```python
from build123d import *

# Parameters (mm, degrees)
SKETCH1_R           = 85
SKETCH1_R_2         = 65
SKETCH1_W           = 2.9
SKETCH1_H           = 40
BOSS_EXTRUDE1_DEPTH = 2.9


with BuildPart() as part:
    # Sketch1 → Boss-Extrude1 (new body)
    with BuildSketch(Plane.XY):
        Circle(SKETCH1_R)
        Circle(SKETCH1_R_2, mode=Mode.SUBTRACT)
        with Locations((-75, 0)):
            Rectangle(SKETCH1_W, SKETCH1_H, mode=Mode.SUBTRACT)
        with Locations((75, 0)):
            Rectangle(SKETCH1_W, SKETCH1_H, mode=Mode.SUBTRACT)
    extrude(amount=BOSS_EXTRUDE1_DEPTH)


solid = part.part
```
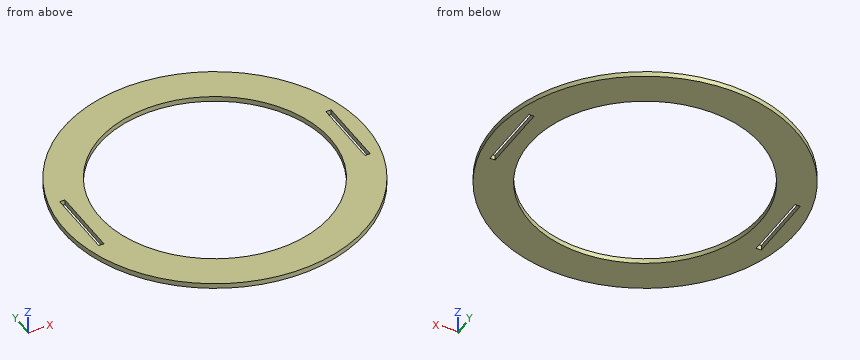
Build history of the part. All positions in model axes, mm. Give positions to 0.01 mm unless a question says otherwise; leave off trailing zeros. Order: outer loops, then holes, each group sorted by start corner. A loop starts at its lowest first (then second) coordinate and runs counter-clockwise, first axis right, second up. Notation, with made-up numbers: M -27,-39.75 L 29,-39.75 A29 cw 29,-6.75 Z; hole C 73.5,16.25 d5. An arc over 180 degrees is marked long. Write item = value, one per line. Start each with the question number.
(1) Pin check, flat tips, straight feed: pin 1 Ø1.5 at (x, z) = (6, 1) entering from -Y; pin 2 Ø0.9 at (y, z) = (-4.5, 2) entering from +X; pin 3 Ø0.9 at (x, z) = (-75.5, 1.5) entering from +Y; pin 4 Ø1.5 at (x, y) = (47.5, 58) entering from -Z. Stop position of each tip, or through.
(2) Probe L1, parallel to X at y = -1.5, z = 2.2; L2, parallel to Y at x = 0, z = 2.6; L3, parallel to Y at x = -59.5, z = 0.4. List the from-to ranges inside material, lowest first. Write a range as [from, to].
(3) Slice it at B-B on z = 2. Write the cut outline in (x, y), plus the area to 3 significant figures.
(4) Slice it at C-C on y = 0. Write the cut outline in (x, z).
(5) Slice it at D-D on y = 27.5. Write the cut outline in (x, z).
(6) Slice it at A-A on x = 0. Write the cut outline in (y, z).
Responses:
q1.pin_1 = -84.84
q1.pin_2 = 84.9
q1.pin_3 = 39.91
q1.pin_4 = 0
q2.L1 = [-84.99, -76.45], [-73.55, -64.98], [64.98, 73.55], [76.45, 84.99]
q2.L2 = [-85, -65], [65, 85]
q2.L3 = [-60.7, -26.17], [26.17, 60.7]
q3.outline = C 0,0 d170; hole M -76.45,-20 L -73.55,-20 L -73.55,20 L -76.45,20 Z; hole C 0,0 d130; hole M 73.55,-20 L 76.45,-20 L 76.45,20 L 73.55,20 Z
q3.area = 9,190 mm2
q4.outline = M -85,0 L -76.45,0 L -76.45,2.9 L -85,2.9 Z; M -73.55,0 L -65,0 L -65,2.9 L -73.55,2.9 Z; M 65,0 L 73.55,0 L 73.55,2.9 L 65,2.9 Z; M 76.45,0 L 85,0 L 85,2.9 L 76.45,2.9 Z
q5.outline = M -80.43,0 L -58.9,0 L -58.9,2.9 L -80.43,2.9 Z; M 58.9,0 L 80.43,0 L 80.43,2.9 L 58.9,2.9 Z
q6.outline = M -85,0 L -65,0 L -65,2.9 L -85,2.9 Z; M 65,0 L 85,0 L 85,2.9 L 65,2.9 Z
